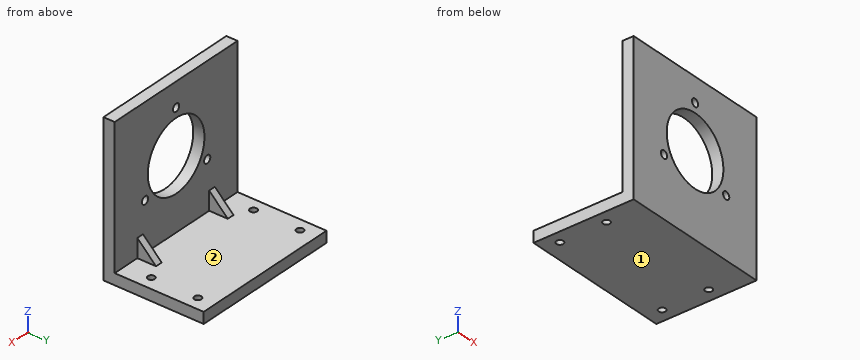
```python
from build123d import *

# Parameters (mm, degrees)
F0_W     = 65
F0_H     = 43
F0_R     = 1.5
F1_DEPTH = 4.8
F3_DEPTH = 59.7
F5_DEPTH = 53.001
F6_R     = 15
F7_DEPTH = 43.001
F8_D     = 3.3


with BuildPart() as f1:
    # F0 (on Top) → F1 (new body)
    with BuildSketch(Plane.XY):
        Rectangle(F0_W, F0_H)
        with Locations((-27.16, -5.5)):
            Circle(F0_R, mode=Mode.SUBTRACT)
        with Locations((26.94, -5.5)):
            Circle(F0_R, mode=Mode.SUBTRACT)
        with Locations((-27.16, 14.5)):
            Circle(F0_R, mode=Mode.SUBTRACT)
        with Locations((26.94, 14.5)):
            Circle(F0_R, mode=Mode.SUBTRACT)
    extrude(amount=F1_DEPTH)

    # F2 (on face) → F3 (join)
    with BuildSketch(Plane.XY.offset(4.8)):
        Polygon((-20.5, -16.7), (-32.5, -16.7), (-32.5, -21.5), (32.5, -21.5), (32.5, -16.7), (20.5, -16.7), (20.5, -8.7), (17.5, -8.7), (17.5, -16.7), (-17.5, -16.7), (-17.5, -8.7), (-20.5, -8.7), align=None)
    extrude(amount=F3_DEPTH)

    # F4 (on face) → F5 (cut, through all)
    with BuildSketch(Plane(origin=(-20.5, 0, 0), x_dir=(0, -1, 0), z_dir=(-1, 0, 0))):
        Polygon((16.7, 12.8), (16.7, 64.5), (8.7, 64.5), (8.7, 4.8), align=None)
    extrude(amount=-F5_DEPTH, mode=Mode.SUBTRACT)

    # F6 (on face) → F7 (cut, through all)
    with BuildSketch(Plane.XZ.offset(21.5)):
        with Locations((0, 35.14)):
            Circle(F6_R)
    extrude(amount=-F7_DEPTH, mode=Mode.SUBTRACT)

    # F8 (through all)
    with Locations(Plane.XZ.offset(21.5)):
        with Locations((0, 54.14), (-16.454483, 25.64), (16.454483, 25.64)):
            Hole(F8_D / 2)


solid = f1.part
```
Model file for the job. Use its own axes, mm. Face numbers are marked on the shaded views. A direction names the side the tool comes from. Coordinates: 2 decimals unless noted, no trailing zeros. Loops run counter-clockwise (first coordinate to the right, second up) from the corner with the lowest first, then second, coordinate; pieces in that order, holes last. Notation, with made-up numbers: (24.5, 33.25) - (55.5, 33.25) arc R9 cw to (55.5, 40.25) - close; hole circle Ø6 at (-22.5, 54). An arc over 180 degrees is marked (long way). Answer as a JSON object with one key per item and string values. Group by question number.
(1) Flat gauge pins, fed straight in: pin 1 (5 mm diameter, centred on x = 26.94, y = 14.5, fed in from +Z); pin 2 (4 mm diameter, centred on y = -13, z = 7.5, fed in from +X); pin 3 (4.5 mm diameter, centred on x = 0, z = 54.14, fed in from +Y); pin 4 (6 mm diameter, centred on x = -11.5, y = -2, fed in from -Z). Where does each tip first touch, or does it go through?
(2) Tool access for the marked faces 1 and 2: list every direction of +Z, -Z, +X, -X, +Y, -Y with a clear straight run to the whole face (end or side of a thin tool).
(3) Probe line 1 along Z through (x, y) = (0, -20); line 2 along Y through (x, z) = (26.94, 1.95); line 3 along Z through (x, y) = (-10, 14). List the from-to ranges inside material, lowest first.
(4) Cut at C-C (y = -5.5). Give the cut face in (x, z), then the cut area to 3 significant figures.
(5) Cut at B-B (x = 26.94). Give the cut face in (y, z), then the cut area to 3 significant figures.
(6) Cut at D-D (z = 7). Give the cut face in (x, y), then the cut area to 3 significant figures.
(7) Cut at A-A (z = 54.14). Give the cut face in (x, y), then the cut area to 3 significant figures.
Geometry says:
{
 "1": {"pin 1": "stops at z = 4.8", "pin 2": "stops at x = 20.5", "pin 3": "stops at y = -16.7", "pin 4": "stops at z = 0"},
 "2": {"face 1": "-Z, +X, -X, +Y, -Y", "face 2": "+Z, +Y"},
 "3": {"line 1": "z = 0 to 20.14, 50.14 to 52.49, 55.79 to 64.5", "line 2": "y = -21.5 to -7, -4 to 13, 16 to 21.5", "line 3": "z = 0 to 4.8"},
 "4": {"outline": "(-32.5, 0) - (-28.66, 0) - (-28.66, 4.8) - (-32.5, 4.8) - close; (-25.66, 0) - (25.44, 0) - (25.44, 4.8) - (-25.66, 4.8) - close; (28.44, 0) - (32.5, 0) - (32.5, 4.8) - (28.44, 4.8) - close", "area": "283 mm^2"},
 "5": {"outline": "(-21.5, 0) - (-7, 0) - (-7, 4.8) - (-16.7, 4.8) - (-16.7, 64.5) - (-21.5, 64.5) - close; (-4, 0) - (13, 0) - (13, 4.8) - (-4, 4.8) - close; (16, 0) - (21.5, 0) - (21.5, 4.8) - (16, 4.8) - close", "area": "464 mm^2"},
 "6": {"outline": "(-32.5, -21.5) - (32.5, -21.5) - (32.5, -16.7) - (20.5, -16.7) - (20.5, -10.9) - (17.5, -10.9) - (17.5, -16.7) - (-17.5, -16.7) - (-17.5, -10.9) - (-20.5, -10.9) - (-20.5, -16.7) - (-32.5, -16.7) - close", "area": "347 mm^2"},
 "7": {"outline": "(-32.5, -21.5) - (-1.65, -21.5) - (-1.65, -16.7) - (-32.5, -16.7) - close; (1.65, -21.5) - (32.5, -21.5) - (32.5, -16.7) - (1.65, -16.7) - close", "area": "296 mm^2"}
}
